```python
from build123d import *

# Parameters (mm, degrees)
SKETCH3_R           = 2.6
BOSS_EXTRUDE1_DEPTH = 7
SKETCH4_W           = 16
SKETCH4_H           = 16
CUT_EXTRUDE1_DEPTH  = 5
SKETCH5_R           = 2
CUT_EXTRUDE2_DEPTH  = 4
CUT_EXTRUDE3_DEPTH  = 26.961509971
SKETCH8_R           = 1.75
CUT_EXTRUDE4_DEPTH  = 20.33907899
SKETCH9_R           = 2.75
SKETCH9_R_2         = 1.75
BOSS_EXTRUDE3_DEPTH = 4


with BuildPart() as part:
    # Sketch3 → Boss-Extrude1 (new body)
    with BuildSketch(Plane.XY):
        with BuildLine():
            Line((-5, 10), (5, 10))
            ThreePointArc((5, 10), (15, 0), (5, -10))
            Line((5, -10), (-5, -10))
            ThreePointArc((-5, -10), (-15, 0), (-5, 10))
        make_face()
        with Locations((1.905, 3.81)):
            Circle(SKETCH3_R, mode=Mode.SUBTRACT)
        with Locations((1.905, -3.81)):
            Circle(SKETCH3_R, mode=Mode.SUBTRACT)
        with Locations((-1.905, 0)):
            Circle(SKETCH3_R, mode=Mode.SUBTRACT)
    extrude(amount=BOSS_EXTRUDE1_DEPTH)

    # Sketch4 → Cut-Extrude1 (cut)
    with BuildSketch(Plane(origin=(0, 0, 0), x_dir=(-1, 0, 0), z_dir=(0, 0, -1))):
        Rectangle(SKETCH4_W, SKETCH4_H)
    extrude(amount=-CUT_EXTRUDE1_DEPTH, mode=Mode.SUBTRACT)

    # Sketch5 → Cut-Extrude2 (cut)
    with BuildSketch(Plane(origin=(0, 0, 0), x_dir=(-1, 0, 0), z_dir=(0, 0, -1))):
        with Locations((-11.5, -2.5)):
            Circle(SKETCH5_R)
        with Locations((-11.5, 2.5)):
            Circle(SKETCH5_R)
    extrude(amount=-CUT_EXTRUDE2_DEPTH, mode=Mode.SUBTRACT)

    # Sketch6 → Cut-Extrude3 (cut, through all)
    with BuildSketch(Plane.XZ.offset(10)):
        Polygon((-5, 2.336923418), (-15, 7), (-15, 0), (-5, 0), align=None)
        Polygon((0.011548444, 0), (-5, 2.336923418), (-5, 0), align=None)
    extrude(amount=-CUT_EXTRUDE3_DEPTH, mode=Mode.SUBTRACT)

    # Sketch8 → Cut-Extrude4 (cut, through all)
    with BuildSketch(Plane(origin=(0.002062624, 0, 0.004423311), x_dir=(-0.9063077870366496, 0, 0.42261826174070033), z_dir=(-0.4226182617407003, 0, -0.9063077870366495))):
        with Locations((12.691121921, 0)):
            Circle(SKETCH8_R)
    extrude(amount=-CUT_EXTRUDE4_DEPTH, mode=Mode.SUBTRACT)

    # Sketch9 → Boss-Extrude3 (add)
    with BuildSketch(Plane(origin=(0.002062624, 0, 0.004423311), x_dir=(-0.9063077870366496, 0, 0.42261826174070033), z_dir=(-0.4226182617407003, 0, -0.9063077870366495))):
        with Locations((12.691121921, 0)):
            Circle(SKETCH9_R)
        with Locations((12.691121921, 0)):
            Circle(SKETCH9_R_2, mode=Mode.SUBTRACT)
    extrude(amount=-BOSS_EXTRUDE3_DEPTH)


solid = part.part
```
Could you check a few things on this model? Use its own coordinates, in mm. A direction names the side the tool comes from. Round coordinates to 2 decimals unless told otherwise and drop trailing zeros. Loops run counter-clockwise (first coordinate to the right, second up) from the corner with the lowest first, then second, coordinate; pieces in that order, holes last. Notation, with made-up numbers: (25.5, -26.5) -> (55.5, -26.5) arc R9 cw to (55.5, -14.5) -> close; hole circle Ø1 at (83.25, 16.25). An arc over 180 degrees is marked (long way). One line per question, with ' | ' between items.
(1) Thinking about a two-plate mould opening in Y: for faces 1 (the face through (9, 1, 0)), 2 (the face through (1.341, -6.348, 5.986)), 3 (the face through (0, 10, 3)), which applies, released by +Y, released by -Y, zero draft, split by the parting line, or undercut?
Model answer:
face 1: zero draft | face 2: undercut | face 3: released by +Y
(2) If I drill on probe 1 along Y at (x, z) = (2.5, 6); probe 2 along Y at (x, z) = (10.75, 2.75); probe 3 along Z at (x, y) = (4.25, 2.5), over which ranges is the centre line in solid material (lowest first)?
Model answer:
probe 1: y = -10 to -6.34, -1.28 to 1.28, 6.34 to 10 | probe 2: y = -8.18 to -4.35, -0.65 to 0.65, 4.35 to 8.18 | probe 3: z = 5 to 7
(3) If we section it at D-D on y = 7.5: List the corners of the cut face in (x, z) for me.
Model answer:
outline: (-11.61, 5.42) -> (-8, 3.74) -> (-8, 5) -> (8, 5) -> (8, 0) -> (11.61, 0) -> (11.61, 7) -> (-11.61, 7) -> close
(4) For pin 1 Ø8.5 at (x, y) = (1.905, -3.81) entering from +Z; pin 2 Ø12 at (x, y) = (-10, 1.5) entering from +Z; pin 3 Ø1.5 at (y, z) = (-7.5, 4) entering from -X; pin 4 Ø3 at (x, y) = (11.5, 2.5) entering from -Z, each with a flat end and sliding along its axis, tell me the tip position at first contact or that it passes through.
Model answer:
pin 1: stops at z = 7 | pin 2: stops at z = 10.16 | pin 3: stops at x = -10.17 | pin 4: stops at z = 4
(5) If we section it at A-A on x = 1.5: List the corners of the cut face in (y, z) for me, and give its area (3 significant figures).
Model answer:
outline: (-10, 0) -> (-8, 0) -> (-8, 5) -> (-6.38, 5) -> (-6.38, 7) -> (-10, 7) -> close; (-1.24, 5) -> (1.24, 5) -> (1.24, 7) -> (-1.24, 7) -> close; (6.38, 5) -> (8, 5) -> (8, 0) -> (10, 0) -> (10, 7) -> (6.38, 7) -> close | area: 39.5 mm^2
(6) For faces 4 (the face through (-9.498, 1.183, 6.61)), 5 (the face through (12, 3, 4)), which set-ups out of +Z, -Z, +X, -X, +Y, -Y let a thin tool reach every point of the face, with its end or its side?
Model answer:
face 4: none | face 5: -Z
(7) If we section it at B-B on y = -5.75: List the corners of the cut face in (x, z) for me, and give its area (3 significant figures).
Model answer:
outline: (-13.18, 6.15) -> (-8, 3.74) -> (-8, 5) -> (0.17, 5) -> (0.17, 7) -> (-13.18, 7) -> close; (3.64, 5) -> (8, 5) -> (8, 0) -> (13.18, 0) -> (13.18, 7) -> (3.64, 7) -> close | area: 72.0 mm^2
(8) If we section it at C-C on z = 3: List the corners of the cut face in (x, y) for me, and give its area (3 significant figures).
Model answer:
outline: (-6.42, -9.9) arc R10 ccw to (-5, -10) -> (5, -10) arc R10 ccw to (5, 10) -> (-5, 10) arc R10 ccw to (-6.42, 9.9) -> (-6.42, 8) -> (8, 8) -> (8, -8) -> (-6.42, -8) -> close; hole circle Ø4 at (11.5, -2.5); hole circle Ø4 at (11.5, 2.5) | area: 130 mm^2
